Part model, mm, in its own coordinate system. A direction names the side the tool comes from. Give positions to 0.01 mm unless a question says otherwise; leave off trailing zeros. Order: outer loops, then holes, each group sorted by start corner. A loop starts at its lowest first (then second) coordinate and runs counter-clockwise, first axis right, second up. Notation, with made-up numbers: (-35, 74.5) - (-18, 74.5) arc R20 ccw to (-18, 91.5) - close; hole circle Ø5 at (69, 35.5). An arc over 180 degrees is marked (long way). Use a Markdown table: item, result. Add a question column.
from build123d import *

# Parameters (mm, degrees)
SKETCH1_R           = 6
BOSS_EXTRUDE1_DEPTH = 3.2
CUT_EXTRUDE1_DEPTH  = 1.8
SKETCH3_R           = 1.6
CUT_EXTRUDE2_DEPTH  = 3.8


with BuildPart() as part:
    # Sketch1 → Boss-Extrude1 (new body)
    with BuildSketch(Plane.XY):
        with Locations((58.8, 0)):
            Circle(SKETCH1_R)
    extrude(amount=BOSS_EXTRUDE1_DEPTH)

    # Sketch2 → Cut-Extrude1 (cut)
    with BuildSketch(Plane.XY.offset(3.2)):
        Polygon((59.35924592, 3.543162701), (56.036154051, 2.212601254), (55.526908131, -1.330561447), (58.34075408, -3.543162701), (61.663845949, -2.212601254), (62.173091869, 1.330561447), align=None)
    extrude(amount=-CUT_EXTRUDE1_DEPTH, mode=Mode.SUBTRACT)

    # Sketch3 → Cut-Extrude2 (cut)
    with BuildSketch(Plane.XY.offset(1.4)):
        with Locations((58.85, 0)):
            Circle(SKETCH3_R)
    extrude(amount=-CUT_EXTRUDE2_DEPTH, mode=Mode.SUBTRACT)


solid = part.part
1. Tool access for faces 4 (the face through (60, 1.4, 0)), 5 (the face through (59.979, -2.887, 2.313)): list every direction of +Z, -Z, +X, -X, +Y, -Y with a clear straight run to the whole face (end or side of a thin tool).
2. Cut at C-C (x = 58.8). Write the cut outline in (y, z).
3. Pin check, flat tips, straight feed: P1, Ø4, axis at x = 57, y = 3.5, coming from the -Z side; P2, Ø3.5, axis at x = 58.85, y = 0, coming from the +Z side; P3, Ø1, axis at x = 57, z = 1.5, coming from the -Y side; P4, Ø1.5, axis at y = 4, z = 2.5, coming from the +X side. Stop position of each tip, or through.
4. Cut at A-A (z = 1.8). Write the cut outline in (x, y).
5. Drill centre lines: probe 1 along Y at (x, z) = (58.85, 0.95); probe 2 along X at (y, z) = (-0.5, 1.25); probe 3 along X at (y, z) = (-1.25, 2.75). Where is each one in solid material? Low to high. Write a range as [from, to].
6. Cut at B-B (y = 0). Write the cut outline in (x, z), plus the area to 3 significant figures.
7. Cut at D-D (y = -2). Write the cut outline in (x, z), plus the area to 3 significant figures.
8. Mould opens along Y. For faces 1 (the face through (61, -3, 3.2)), 2 (the face through (52.806, 0.264, 1.578)), 3 (the face through (56.91, -2.42, 2.31)) say: released by +Y, released by -Y, zero draft, split by the parting line, or undercut.
Responses:
| question | item | result |
|---|---|---|
| 1 | face 4 | -Z, +X, -X, +Y, -Y |
| 1 | face 5 | +Z |
| 2 | outline | (-6, 0) - (-1.6, 0) - (-1.6, 1.4) - (-3.36, 1.4) - (-3.36, 3.2) - (-6, 3.2) - close; (1.6, 0) - (6, 0) - (6, 3.2) - (3.32, 3.2) - (3.32, 1.4) - (1.6, 1.4) - close |
| 3 | P1 | stops at z = 0 |
| 3 | P2 | stops at z = 1.4 |
| 3 | P3 | stops at y = -5.86 |
| 3 | P4 | stops at x = 63.84 |
| 4 | outline | circle Ø12 at (58.8, 0); hole (55.53, -1.33) - (58.34, -3.54) - (61.66, -2.21) - (62.17, 1.33) - (59.36, 3.54) - (56.04, 2.21) - close |
| 5 | probe 1 | y = [-6, -1.6], [1.6, 6] |
| 5 | probe 2 | x = [52.82, 57.33], [60.37, 64.78] |
| 5 | probe 3 | x = [52.93, 55.54], [61.8, 64.67] |
| 6 | outline | (52.8, 0) - (57.25, 0) - (57.25, 1.4) - (55.72, 1.4) - (55.72, 3.2) - (52.8, 3.2) - close; (60.45, 0) - (64.8, 0) - (64.8, 3.2) - (61.98, 3.2) - (61.98, 1.4) - (60.45, 1.4) - close |
| 6 | area | 22.6 mm² |
| 7 | outline | (53.14, 0) - (64.46, 0) - (64.46, 3.2) - (61.69, 3.2) - (61.69, 1.4) - (56.38, 1.4) - (56.38, 3.2) - (53.14, 3.2) - close |
| 7 | area | 26.6 mm² |
| 8 | face 1 | zero draft |
| 8 | face 2 | split by the parting line |
| 8 | face 3 | undercut |
